Verification items for the finished model (mm, model axes). A direction names the side the tool comes from. Round coordinates to 2 decimals unless told otherwise and drop trailing zeros. Order: outer loops, then holes, each group sorted by start corner. A loop starts at its lowest first (then second) coordinate and runs counter-clockwise, first axis right, second up. Notation, with made-up numbers: (70.25, 4) -> (81.25, 4) arc R11 cw to (81.25, 16) -> close; hole circle Ø9 at (50.5, 58.25). An arc over 180 degrees is marked (long way). Return JSON: item names as keys, results as strings. Group by question number.
Item 1: Sectioned sample at B-B on z = 8.35. Record the cut outline in (x, y).
Item 2: Scan lines: probe 1 along Y at (x, z) = (0.5, 2.5); probe 2 along Z at (x, y) = (3.75, 2); probe 3 along Z at (x, y) = (4.5, 4). Record each from-to range of solid material in increasing order. Write a range as from..to.
Item 3: Sectioned sample at C-C on y = 6.75. Record the cut outline in (x, z), plus the area to 3 significant figures.
Item 4: Sectioned sample at A-A on x = 2.5. Give the number of separate pieces and of enclosed holes in the cut face, plus the area to 3 significant figures.
Item 5: Draft check along Z on faces 3 (the flat face through (6.35, 2, 8)), 4 (the cylindrical face through (4.674, 2.492, 15.809)), 5 (the flat face through (3, 9, 6.35)). Enter one of: pulls with the +Z half, pulls with the -Z half, needs draft (parallel to the pull), parting line crosses it, or undercut.
Item 6: Access from +Z, -Z, +X, -X, +Y, -Y to the whole of each face (thin tool, end or side, straight path). Record for faces 1 (the flat face through (3, 5.08, 14)), 2 (the cylindrical face through (3.23, 1.71, 3.5)).
Item 7: Depth check by flat-ended pin: pin 1 Ø1.5 at (x, y) = (2.5, 10) entering from +Z; pin 2 Ø5 at (y, z) = (9.525, 3.175) entering from +X; pin 3 Ø3 at (x, z) = (3, 13.5) entering from +Y; pin 4 Ø1 at (x, z) = (4.5, 7.5) entering from +Y. Enter the tip coordinate at first touch or a pass-through.
```python
from build123d import *

# Parameters (mm, degrees)
BOSS_EXTRUDE1_DEPTH             = 6.35
F_3_0MM_DOWEL_HOLE1_D           = 3
F_3_0MM_DOWEL_HOLE1_CSINK_D     = 3.05
F_3_0MM_DOWEL_HOLE1_CSINK_ANGLE = 90
F_3_0MM_DOWEL_HOLE2_D           = 3
F_3_0MM_DOWEL_HOLE2_CSINK_D     = 3.05
F_3_0MM_DOWEL_HOLE2_CSINK_ANGLE = 90


with BuildPart() as part:
    # Sketch1 → Boss-Extrude1 (new body)
    with BuildSketch(Plane(origin=(0, 0, 0), x_dir=(0, 0, -1), z_dir=(1, 0, 0))):
        with BuildLine():
            Line((-19.05, 0), (0, 0))
            Line((0, 0), (0, 12.7))
            Line((0, 12.7), (-6.35, 12.7))
            Line((-6.35, 12.7), (-6.35, 5.08))
            ThreePointArc((-6.35, 5.08), (-8.35, 3.08), (-10.35, 5.08))
            Line((-10.35, 5.08), (-19.05, 5.08))
            Line((-19.05, 5.08), (-19.05, 0))
        make_face()
    extrude(amount=BOSS_EXTRUDE1_DEPTH)

    # Ø3.0mm Dowel Hole1 (through all)
    with Locations(Plane.ZY):
        with Locations((3.175, 3.175), (3.175, 9.525)):
            CounterSinkHole(F_3_0MM_DOWEL_HOLE1_D / 2, F_3_0MM_DOWEL_HOLE1_CSINK_D / 2, counter_sink_angle=F_3_0MM_DOWEL_HOLE1_CSINK_ANGLE)

    # Ø3.0mm Dowel Hole2 (through all)
    with Locations(Plane(origin=(0, 5.08, 0), x_dir=(1, 0, 0), z_dir=(0, 1, 0))):
        with Locations((3.175, -15.875)):
            CounterSinkHole(F_3_0MM_DOWEL_HOLE2_D / 2, F_3_0MM_DOWEL_HOLE2_CSINK_D / 2, counter_sink_angle=F_3_0MM_DOWEL_HOLE2_CSINK_ANGLE)


solid = part.part
```
Recorded:
{
 "1": {"outline": "(0, 0) -> (6.35, 0) -> (6.35, 3.08) -> (0, 3.08) -> close"},
 "2": {"probe 1": "0..1.84, 4.51..8.19, 10.86..12.7", "probe 2": "0..2.24, 4.11..14.49, 17.26..19.05", "probe 3": "0..1.92, 4.43..6.67, 10.03..15.17, 16.58..19.05"},
 "3": {"outline": "(0, 0) -> (6.35, 0) -> (6.35, 6.35) -> (0, 6.35) -> close", "area": "40.3 mm²"},
 "4": {"separate pieces": "2", "enclosed holes": "2", "area": "111 mm²"},
 "5": {"face 3": "needs draft", "face 4": "undercut", "face 5": "pulls with the +Z half"},
 "6": {"face 1": "+Z, +X, -X, +Y", "face 2": "+X, -X"},
 "7": {"pin 1": "z = 6.35", "pin 2": "x = 6.35", "pin 3": "y = 5.08", "pin 4": "y = 3.6"}
}
